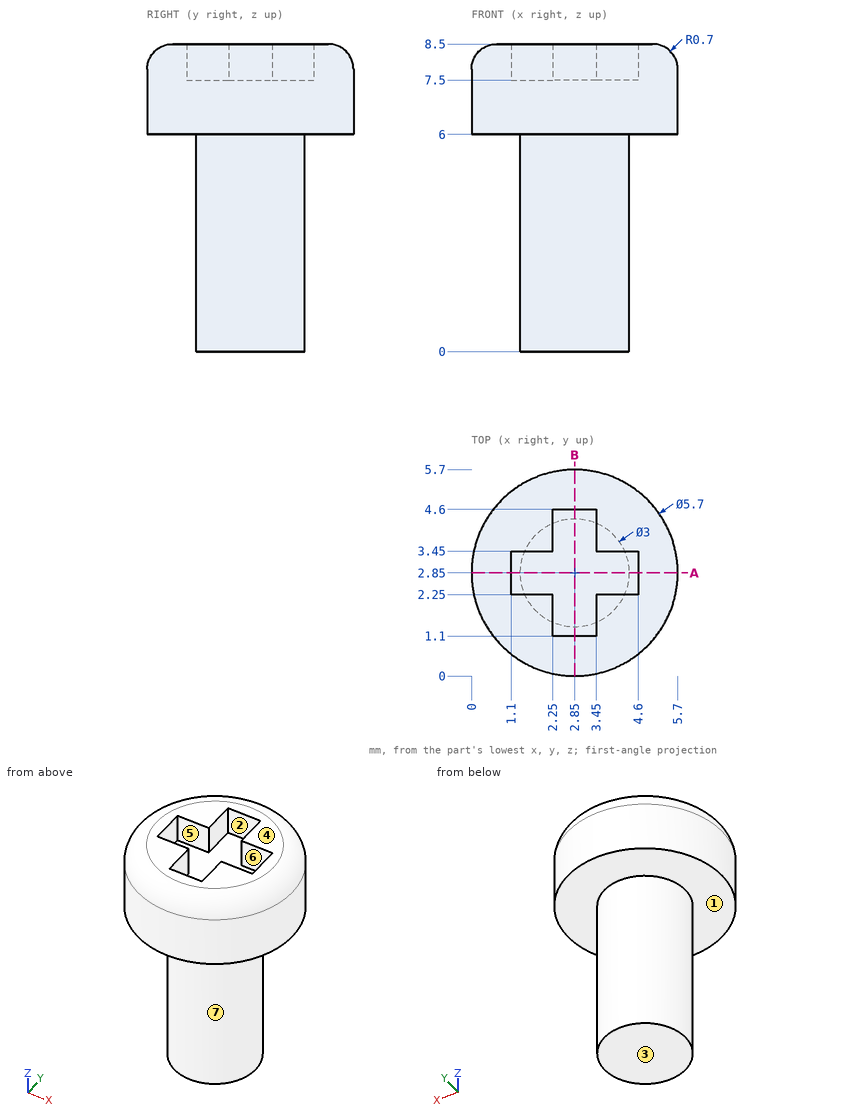
Geometry: see drawing. Coordinates: mm, zero at the bounding-box minimum. A direction names the side the tool comes from. Round coordinates to 2 decimals unless told otherwise and drop trailing zeros. Write each loop counter-clockwise with the first axis right and the second up, starting at its lowest first coordinate (ties: lowest second). Pieces come first, ordered by that corner, then holes.
1) Reachability of the marked faces 1, 2 and 3 from +Z, -Z, +X, -X, +Y, -Y: full face, straight path, thin tool, end or side. Return the list, or none.
2) Draft query along Y for the marked faces 4, 5, 6 and 7. Return one class per face: pulls with the +Y half, pulls with the -Y half, needs draft (parallel to the pull), parting line crosses it, or undercut.
3) Ray query, L1, parallel to Z at x = 4.1, y = 3.8; L2, parallel to Z at x = 1.75, y = 3.4; L3, parallel to X at y = 1.8, z = 8.25. Return the intervals inside material, ascending.
4) Contact query for flat-ended pins moving along their axis: P1, Ø1.5, axis at y = 4.5, z = 2, coming from the -X side; P2, Ø0.8, axis at y = 4, z = 8, coming from the -X side; P3, Ø3, axis at x = 2.5, z = 2.5, coming from the +Y side. Output: stop coordinate, or through.
5) Cut plane A-A (y = 2.85). Return the cut outline in (x, z), then the cut area to 3 significant figures.
Geometry says:
1. face 1: -Z
1. face 2: +Z
1. face 3: -Z, +X, -X, +Y, -Y
2. face 4: needs draft
2. face 5: undercut
2. face 6: undercut
2. face 7: parting line crosses it
3. L1: z = 6 to 8.5
3. L2: z = 0 to 7.5
3. L3: x = 0.38 to 2.25, 3.45 to 5.32
4. P1: stops at x = 1.65
4. P2: stops at x = 0.11
4. P3: stops at y = 4.35
5. outline: (0, 6) - (1.35, 6) - (1.35, 0) - (4.35, 0) - (4.35, 6) - (5.7, 6) - (5.7, 7.8) arc R0.7 ccw to (5, 8.5) - (4.6, 8.5) - (4.6, 7.5) - (1.1, 7.5) - (1.1, 8.5) - (0.7, 8.5) arc R0.7 ccw to (0, 7.8) - close
5. area: 28.5 mm2
